Autodesk Inventor part; units mm, degrees
ref_plane "YZ Plane" through (0, 0, 0) normal (1, 0, 0) x (0, 1, 0)
ref_plane "XZ Plane" through (0, 0, 0) normal (0, 1, 0) x (-1, 0, 0)
ref_plane "XY Plane" through (0, 0, 0) normal (0, 0, 1) x (1, 0, 0)
sketch "Sketch1" plane through (0, 0, 0) normal (0, 1, 0) x (-1, 0, 0)
  line L0 (-0.7821, 21.3445) -> (84.5093, 28.8066)
  line L1 (84.5093, 28.8066) -> (84.5093, 40.7189)
  arc A0 (84.5093, 40.7189) -> (70.3763, 53.6694) centre (71.5093, 40.7189) ccw
  line L2 (70.3763, 53.6694) -> (-16.1101, 46.1028)
  line L3 (-16.1101, 46.1028) -> (-16.1101, 35.3901)
  line L4 (-16.1101, 35.3901) -> (-0.7821, 21.3445)
  line L5 (82.5093, 40.7189) -> (82.5093, 35.2209)
  arc A1 (77.9451, 30.2399) -> (82.5093, 35.2209) centre (77.5093, 35.2209) ccw
  line L6 (77.9451, 30.2399) -> (2.112, 23.6054)
  arc A2 (-1.7018, 24.8999) -> (2.112, 23.6054) centre (1.6762, 28.5863) ccw
  line L7 (-1.7018, 24.8999) -> (-12.4881, 34.7838)
  arc A3 (-14.1101, 38.4702) -> (-12.4881, 34.7838) centre (-9.1101, 38.4702) ccw
  line L8 (-14.1101, 38.4702) -> (-14.1101, 39.6885)
  arc A4 (-9.5459, 44.6695) -> (-14.1101, 39.6885) centre (-9.1101, 39.6885) ccw
  line L9 (-9.5459, 44.6695) -> (70.5506, 51.677)
  arc A5 (82.5093, 40.7189) -> (70.5506, 51.677) centre (71.5093, 40.7189) ccw
  line L10 (-15.9101, 45.9195) -> (70.3937, 53.4702)
  arc A6 (84.3093, 40.7189) -> (70.3937, 53.4702) centre (71.5093, 40.7189) ccw
  line L11 (84.3093, 40.7189) -> (84.3093, 28.9898)
  line L12 (84.3093, 28.9898) -> (-0.7118, 21.5514)
  line L13 (-0.7118, 21.5514) -> (-15.9101, 35.4781)
  line L14 (-15.9101, 35.4781) -> (-15.9101, 45.9195)
  point P0 (0, 0)
  dimension "d0" = 0.2
extrude "Extrusion1" add sketch "Sketch1" along normal blind 0.4 contours L4 L3 L2 A0 L1 L0 | L5 A1 L6 A2 L7 A3 L8 A4 L9 A5 | L10 A6 L11 L12 L13 L14
properties part number "e"
Could you check a few things on this model? Use its own coordinates, in mm. Give positions to 0.01 mm unless a question says otherwise; leave off trailing zeros. Write each loop counter-clockwise with the first axis right and the second up, starting at its lowest first coordinate (ties: lowest second). Pieces come first, ordered by that corner, then holes. Notation, with made-up numbers: (27, 54.25) - (33, 54.25) arc R31 cw to (33, 78.25) - close; hole circle Ø6 at (41.5, -31.5). An arc over 180 degrees is marked (long way). Use CSV: the item, a comma, the result in double quotes. Start each with the question number.
Item 1: I want a section at B-B, the plane z = 27.5. Please give me the cut outline in (x, y), then the cut area to 3 significant figures.
Item 2: I want a section at A-A, the plane y = 0.15. Please give me the cut outline in (x, z), then the cut area to 3 significant figures.
Item 3: If I drill on line 1 along Z through (x, y) = (-3, 0.1); line 2 along X through (y, z) = (0.2, 30); line 3 along X through (y, z) = (0.15, 42), over which ranges is the centre line in solid material (lowest first)?
Item 4: I want a section at C-C, the plane x = -39. Please give me the cut outline in (y, z).
Findings:
1,outline,"(-69.57, 0) - (7.5, 0) - (7.5, 0.4) - (-69.57, 0.4) - close"
1,area,"30.8 mm2"
2,outline,"(-84.51, 28.81) - (0.78, 21.34) - (16.11, 35.39) - (16.11, 46.1) - (-70.38, 53.67) arc R13 ccw to (-84.51, 40.72) - close"
2,area,"2,460 mm2"
3,line 1,"z = 21.68 to 47.77"
3,line 2,"x = -84.51 to 10.23"
3,line 3,"x = -84.45 to 16.11"
4,outline,"(0, 24.83) - (0.4, 24.83) - (0.4, 50.92) - (0, 50.92) - close"
